Can you work these out from the model? Positions are in its coordinate system, mm. A direction names the side the tool comes from. Round coordinates to 2 decimals unless told otherwise and drop trailing zeros. Loops run counter-clockwise (first coordinate to the right, second up) from the corner with the lowest first, then second, coordinate; pieces in that order, holes last. Notation, with made-up numbers: M 65.25,41.5 L 76.25,41.5 A20 cw 76.25,75.5 Z; hole C -16.5,49 d3. An arc over 180 degrees is marked long. Use a Markdown table: item, result. Add a question column.
Autodesk Inventor part; units mm, degrees
ref_plane "YZ Plane" through (0, 0, 0) normal (1, 0, 0) x (0, 1, 0)
ref_plane "XZ Plane" through (0, 0, 0) normal (0, 1, 0) x (-1, 0, 0)
ref_plane "XY Plane" through (0, 0, 0) normal (0, 0, 1) x (1, 0, 0)
sketch "スケッチ1" plane through (0, 0, 0) normal (0, 0, 1) x (1, 0, 0)
  circle A0 centre (250, 70) radius 2.1 construction
  circle A1 centre (250, 85) radius 2.1 construction
  line L0 (258.724, 99.45) -> (245, 99.45)
  arc A2 (245, 70) -> (250, 65) centre (250, 70) ccw
  line L1 (245, 70) -> (245, 99.45)
  line L2 (258.724, 99.45) -> (258.724, 65)
  line L3 (258.724, 65) -> (250, 65)
  circle A3 centre (250, 70) radius 2.25
  circle A4 centre (250, 85) radius 2.25
  point P0 (0, 0)
  dimension "d0" = 4.5
extrude "押し出し1" add sketch "スケッチ1" along normal blind 7
sketch "スケッチ2" plane through (245, 99.45, 0) normal (0, 1, 0) x (1, 0, 0)
  circle A0 centre (5, -3.5) radius 1.65 construction
  circle A1 centre (5, -3.5) radius 2.25
  point P0 (-245, 0)
  dimension "d3" = 4.5
extrude "押し出し2" cut sketch "スケッチ2" against normal blind 6
properties part number "pci_slot_adapter_04"
(1) Suppose I cut it at C-C on y = 94. List the corners of the cut face in (x, z) for me, and give its area (3 significant figures).
(2) Suppose I cut it at A-A on y = 85. List the corners of the cut face in (x, z) for me, and give its area (3 significant figures).
(3) If I drill on probe 1 along Y at (x, z) = (250, 4); probe 2 along X at (y, z) = (95.15, 3.5); probe 3 along X at (y, z) = (72, 6.5), over which ranges is the centre line in solid material (lowest first)? Write a range as [from, to].
(4) Suppose I cut it at B-B on z = 3.5. List the corners of the cut face in (x, y) for me.
(5) Thinking about a two-plate mould opening in X: for faces 3 (the face through (245, 85, 3)), 4 (the face through (248.214, 71.369, 3.451)), 5 (the face through (258.724, 82, 3)), which applies, released by +X, released by -X, zero draft, split by the parting line, or undercut?
(6) On a 3-axis mill with a long thin cutter (end or side, diameter ignored), from which of +Z, -Z, +X, -X, +Y, -Y can I reach the whole of each face in a straight line? I mean faces 1 (the face through (252, 82, 0)), 2 (the face through (247.752, 96.492, 3.401)). Say none if no direction works.
(7) I'm going to push a flat-ended pin straight in: pin 1 (2.5 mm diameter, centred on x = 250, z = 3.5, fed in from +Y). Where does the tip first touch, or does it pass through?
Results below:
| question | item | result |
|---|---|---|
| 1 | outline | M 245,0 L 258.72,0 L 258.72,7 L 245,7 Z; hole C 250,3.5 d4.5 |
| 1 | area | 80.2 mm² |
| 2 | outline | M 245,0 L 247.75,0 L 247.75,7 L 245,7 Z; M 252.25,0 L 258.72,0 L 258.72,7 L 252.25,7 Z |
| 2 | area | 64.6 mm² |
| 3 | probe 1 | y = [65, 67.75], [72.25, 82.75], [87.25, 93.45] |
| 3 | probe 2 | x = [245, 247.75], [252.25, 258.72] |
| 3 | probe 3 | x = [245, 248.97], [251.03, 258.72] |
| 4 | outline | M 245,70 A5 ccw 250,65 L 258.72,65 L 258.72,99.45 L 252.25,99.45 L 252.25,93.45 L 247.75,93.45 L 247.75,99.45 L 245,99.45 Z; hole C 250,70 d4.5; hole C 250,85 d4.5 |
| 5 | face 3 | released by -X |
| 5 | face 4 | undercut |
| 5 | face 5 | released by +X |
| 6 | face 1 | -Z, +X, -X, +Y, -Y |
| 6 | face 2 | +Y |
| 7 | pin 1 | stops at y = 93.45 |
